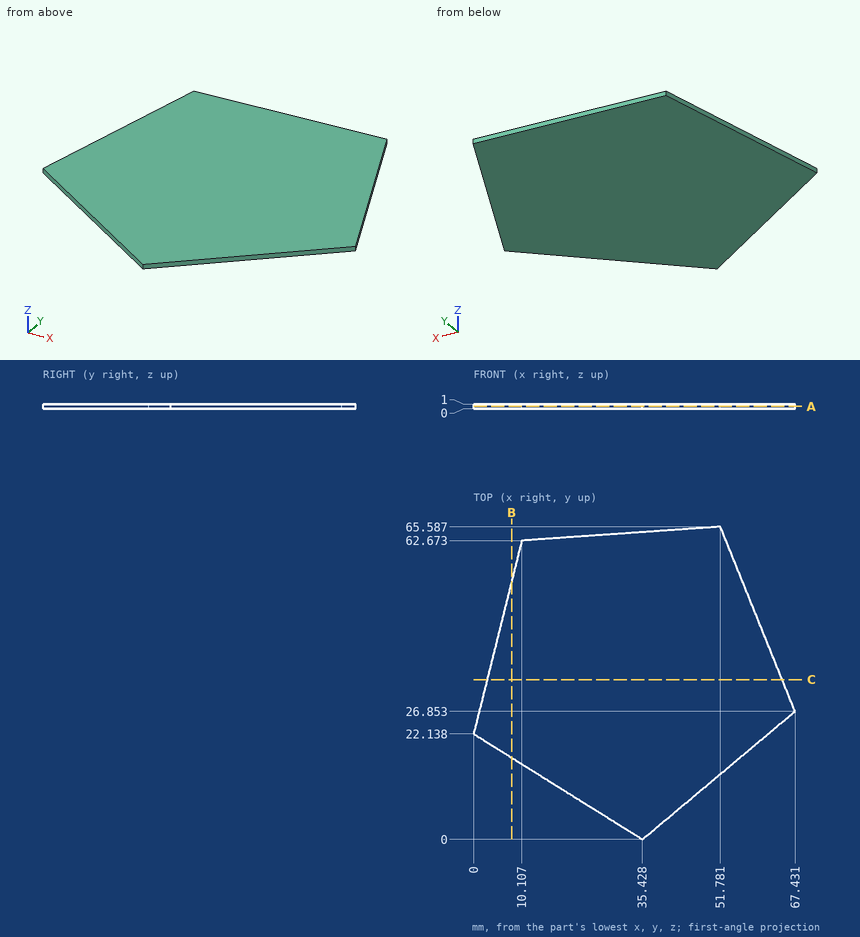
Geometry: see drawing. Coordinates: mm, zero at the bounding-box minimum. Round coordinates to 2 decimals unless told otherwise and drop trailing zeros. Loops run counter-clockwise (first coordinate to the right, second up) from the corner with the lowest first, then second, coordinate; pieces in that order, holes last. Notation, with made-up numbers: (-30, -13.5) -> (0, -13.5) arc R9 cw to (0, -8.5) -> close; hole circle Ø5 at (10, -28.5). An arc over 180 degrees is marked (long way). Use one line per item in the form item = value. Start each with the question number.
Item 1: Section query A-A on z = 0.5. Return the cut outline in (x, y), then the cut area to 3 significant figures.
Item 2: Section query B-B on x = 8. Return the cut outline in (y, z).
Item 3: Material intervals for L1, parallel to Y at x = 23, z = 0.3 (1 decimal); L2, parallel to Y at x = 26, z = 0.8 (1 decimal); L3, parallel to X at y = 29, z = 0.85, sorted ascending. Write a range as from..to.
Item 4: Section query C-C on y = 33.5. Return the cut outline in (x, z) (1 decimal).
Ans:
q1.outline = (0, 22.14) -> (35.43, 0) -> (67.43, 26.85) -> (51.78, 65.59) -> (10.11, 62.67) -> close
q1.area = 3,000 mm^2
q2.outline = (17.14, 0) -> (54.22, 0) -> (54.22, 1) -> (17.14, 1) -> close
q3.L1 = 7.8..63.6
q3.L2 = 5.9..63.8
q3.L3 = 1.71..66.56
q4.outline = (2.8, 0) -> (64.7, 0) -> (64.7, 1) -> (2.8, 1) -> close
